Autodesk Inventor part; units mm, degrees
ref_plane "YZ Plane" through (0, 0, 0) normal (1, 0, 0) x (0, 1, 0)
ref_plane "XZ Plane" through (0, 0, 0) normal (0, 1, 0) x (-1, 0, 0)
ref_plane "XY Plane" through (0, 0, 0) normal (0, 0, 1) x (1, 0, 0)
sketch "Sketch1" plane through (0, 0, 0) normal (1, 0, 0) x (0, 1, 0)
  arc A0 (16.4511, -26.4081) -> (-13.5489, -39.4081) centre (16.4011, -67.4081) ccw
  line L0 (22.4511, -26.4081) -> (16.4511, -26.4081)
  line L1 (-13.5489, 77.5919) -> (-13.5489, -39.4081)
  line L2 (-10.5489, 77.5919) -> (-10.5489, -32.6274)
  arc A1 (16.4529, -23.4081) -> (-10.5489, -32.6274) centre (16.4011, -67.4081) ccw
  line L3 (16.4529, -23.4081) -> (22.4511, -23.4081)
  line L4 (-10.5489, 77.5919) -> (-13.5489, 77.5919)
  line L5 (22.4511, -23.4081) -> (22.4511, -26.4081)
  dimension "d0" = 3
extrude "Extrusion1" add sketch "Sketch1" along normal blind 94
sketch "Sketch2" plane through (0, 0, 0) normal (-1, 0, 0) x (0, 0, 1)
  line L0 (-32.6274, -10.5489) -> (77.5919, -10.5489)
  arc A0 (-32.6274, -10.5489) -> (-23.4081, 16.4529) centre (-67.4081, 16.4011) ccw
  line L1 (-23.4081, 22.4511) -> (-23.4081, 16.4529)
  line L2 (-26.4081, 22.4511) -> (-23.4081, 22.4511)
  line L3 (-26.4081, 16.4511) -> (-26.4081, 22.4511)
  arc A1 (-39.4081, -13.5489) -> (-26.4081, 16.4511) centre (-67.4081, 16.4011) ccw
  line L4 (77.5919, -13.5489) -> (-39.4081, -13.5489)
  line L5 (77.5919, -10.5489) -> (77.5919, -13.5489)
  line L6 (77.5919, -10.5489) -> (57.5919, -10.5489)
  line L7 (57.5919, -10.5489) -> (37.5919, -10.5489)
  line L8 (37.5919, -10.5489) -> (17.5919, -10.5489)
  line L9 (17.5919, -10.5489) -> (-2.4081, -10.5489)
  line L10 (-2.4081, -10.5489) -> (-22.4081, -10.5489)
  line L11 (-22.4081, -10.5489) -> (-22.4081, -13.5489)
  line L12 (-2.4081, -10.5489) -> (-2.4081, -13.5489)
  line L13 (17.5919, -10.5489) -> (17.5919, -13.5489)
  line L14 (37.5919, -10.5489) -> (37.5919, -13.5489)
  line L15 (57.5919, -10.5489) -> (57.5919, -13.5489)
  line L16 (77.5919, -13.5489) -> (-22.4081, -13.5489)
  line L17 (77.5919, -10.5489) -> (-22.4081, -10.5489)
  dimension "d3" = 20
  dimension "d4" = 20
  dimension "d5" = 20
  dimension "d6" = 20
  dimension "d7" = 20
extrude "Extrusion2" cut sketch "Sketch2" against normal blind 3 contours L0 L12 L4 L11 | L0 L14 L4 L13 | L0 L5 L4 L15
sketch "Sketch3" plane through (94, 0, 0) normal (1, 0, 0) x (0, 0, -1)
  line L0 (32.6274, -10.5489) -> (-77.5919, -10.5489)
  line L1 (-77.5919, -10.5489) -> (-77.5919, -13.5489)
  line L2 (-77.5919, -13.5489) -> (39.4081, -13.5489)
  arc A0 (26.4081, 16.4511) -> (39.4081, -13.5489) centre (67.4081, 16.4011) ccw
  line L3 (26.4081, 16.4511) -> (26.4081, 22.4511)
  line L4 (26.4081, 22.4511) -> (23.4081, 22.4511)
  line L5 (23.4081, 22.4511) -> (23.4081, 16.4529)
  arc A1 (23.4081, 16.4529) -> (32.6274, -10.5489) centre (67.4081, 16.4011) ccw
  line L6 (-77.5919, -13.5489) -> (-57.5919, -13.5489)
  line L7 (-57.5919, -13.5489) -> (-37.5919, -13.5489)
  line L8 (-37.5919, -13.5489) -> (-17.5919, -13.5489)
  line L9 (-17.5919, -13.5489) -> (2.4081, -13.5489)
  line L10 (2.4081, -13.5489) -> (22.4081, -13.5489)
  line L11 (22.4081, -13.5489) -> (22.4081, -10.5489)
  line L12 (2.4081, -13.5489) -> (2.4081, -10.5489)
  line L13 (-17.5919, -13.5489) -> (-17.5919, -10.5489)
  line L14 (-37.5919, -13.5489) -> (-37.5919, -10.5489)
  line L15 (-57.5919, -10.5489) -> (-57.5919, -13.5489)
  line L16 (-77.5919, -10.5489) -> (22.4081, -10.5489)
  line L17 (-77.5919, -13.5489) -> (22.4081, -13.5489)
  dimension "d10" = 20
  dimension "d11" = 20
  dimension "d12" = 20
  dimension "d13" = 20
  dimension "d14" = 20
extrude "Extrusion3" cut sketch "Sketch3" against normal blind 3 contours L11 L2 L12 L0 | L13 L2 L14 L0 | L15 L2 L1 L0
sketch "Sketch4" plane through (0, 22.4511, -23.4081) normal (0, 1, 0) x (1, 0, 0)
  line L0 (0, 3) -> (0, 0)
  line L1 (0, 0) -> (94, 0)
  line L2 (94, 3) -> (94, 0)
  line L3 (0, 3) -> (94, 3)
  line L4 (94, 3) -> (0, 3)
  line L5 (94, 3) -> (67, 3)
  line L6 (67, 3) -> (55, 3)
  line L7 (55, 3) -> (43, 3)
  line L8 (43, 3) -> (31, 3)
  line L9 (31, 3) -> (19, 3)
  line L10 (19, 3) -> (0, 3)
  line L11 (67, 3) -> (47, 3)
  line L12 (47, 3) -> (67, 3)
  line L13 (47, 3) -> (27, 3)
  line L14 (94, 3) -> (77, 3)
  line L15 (77, 3) -> (57, 3)
  line L16 (57, 3) -> (37, 3)
  line L17 (37, 3) -> (17, 3)
  line L18 (17, 3) -> (17, 0)
  line L19 (37, 3) -> (37, 0)
  line L20 (57, 3) -> (57, 0)
  line L21 (77, 3) -> (77, 0)
  line L22 (0, 0) -> (0, 3)
  line L23 (94, 0) -> (94, 3)
  line L24 (94, 0) -> (0, 0)
  line L25 (94, 3) -> (0, 3)
  dimension "d26" = 17
  dimension "d27" = 20
  dimension "d28" = 20
  dimension "d29" = 20
extrude "Extrusion4" add sketch "Sketch4" along normal blind 3 contours L3 L18 L1 L0 | L19 L3 L20 L1 | L21 L3 L2 L1
fillet "Fillet1" radius 5 1 edges at (47, -10.5489, -32.6274)
properties part number "bridge plate"
The model under review builds one solid part; all positions refer to its coordinate system, in mm. A direction names the side the tool comes from. Give positions to 0.01 mm unless a question says otherwise; leave off trailing zeros. Order: outer loops, then holes, each group sorted by start corner. A loop starts at its lowest first (then second) coordinate and runs counter-clockwise, first axis right, second up. Notation, with made-up numbers: M 10.25,75 L 64.25,75 A14 cw 64.25,82 Z; hole C 72.5,16.5 d3. An arc over 180 degrees is marked long. One line per question, with ' | ' between items. Start each with the question number.
1) Clearance check with flat-ended pins moving along their axes: P1, Ø2.5, axis at y = -11.5, z = 29.5, coming from the -X side; P2, Ø0.9, axis at x = 92, y = -12.5, coming from the +Z side; P3, Ø0.9, axis at x = 92.5, y = -11.5, coming from the -Z side; P4, Ø3, axis at y = -7.5, z = 55.5, coming from the +X side. State where each tip first meets the part, or that it passes through.
2) Consider section B-B, the plane y = 19.5. Give the boundary of the cut face in (x, z).
3) Consider section A-A, the plane x = 50. Give the boundary of the cut face in (y, z).
4) Consider section C-C, the plane z = 21.5. Give the boundary of the cut face in (x, y), then the cut area to 3 significant figures.
5) For faces 1 (the face through (91, -12, 28)), 2 (the face through (17, 24, -25)), 3 (the face through (93, -12, 57.592)), 4 (the face through (3, -12, -13)), 5 (the face through (46.342, 6.16, -24.617)), list the 3-axis set-ups (+Z, -Z, +X, -X, +Y, -Y) from which the entire face can be reached by the end or side of a thin tool; tool diameter is ignored.
6) Consider section D-D, the plane x = 22.5. Give the boundary of the cut face in (y, z), then the cut area to 3 significant figures.
7) Mouldability with a two-part tool opening along Z and no side actions: class faces 6 (the face through (27, 22.451, -25)), 7 (the face through (47.658, -8.236, -27.816)), 8 (the face through (93, -12, -2.408)) as pulls with the +Z half, pulls with the -Z half, needs draft (parallel to the pull), parting line crosses it, or undercut.
8) Wall thickness on L1, parallel to Y at x = 83, z = -12.5; L2, parallel to Z at x = 90, y = 18.5; L3, parallel to Z at x = 19.5, y = 6.5: over which ranges is each line inside the solid? List them lowest first. Write a range as from..to.
Found:
1) P1: stops at x = 3 | P2: stops at z = 57.59 | P3: stops at z = -37.79 | P4: passes through
2) outline: M 0,-26.41 L 94,-26.41 L 94,-23.41 L 0,-23.41 Z
3) outline: M -13.55,-39.41 A41 cw 16.45,-26.41 L 25.45,-26.41 L 25.45,-23.41 L 16.45,-23.41 A44 ccw -3.31,-28.07 A5 cw -10.55,-23.6 L -10.55,77.59 L -13.55,77.59 Z
4) outline: M 3,-13.55 L 91,-13.55 L 91,-10.55 L 3,-10.55 Z | area: 264 mm²
5) face 1: +X, +Y, -Y | face 2: +Z, -Z, +Y | face 3: +Z, +X, +Y, -Y | face 4: -X, +Y, -Y | face 5: +Z, +X, -X
6) outline: M -13.55,-39.41 A41 cw 16.45,-26.41 L 22.45,-26.41 L 22.45,-23.41 L 16.45,-23.41 A44 ccw -3.31,-28.07 A5 cw -10.55,-23.6 L -10.55,77.59 L -13.55,77.59 Z | area: 469 mm²
7) face 6: needs draft | face 7: pulls with the +Z half | face 8: undercut
8) L1: y = -13.55..-10.55 | L2: z = -26.41..-23.41 | L3: z = -27.62..-24.54
